Print and shaded views of the part. All mm, measured from the part's lowest x, y and z. Give positions to 0.01 mm unless a question says otherwise; leave off trailing zeros. Loops run counter-clockwise (first coordinate to the right, second up) from the corner with the lowest first, then second, coordinate; pieces in that order, holes last. Notation, with made-up numbers: (7.5, 79.5) - (12.5, 79.5) arc R24 cw to (12.5, 118.5) - close; hole circle Ø10 at (66.5, -38.75). An arc over 180 degrees is marked (long way). Return JSON: item names as keys, results as strings.
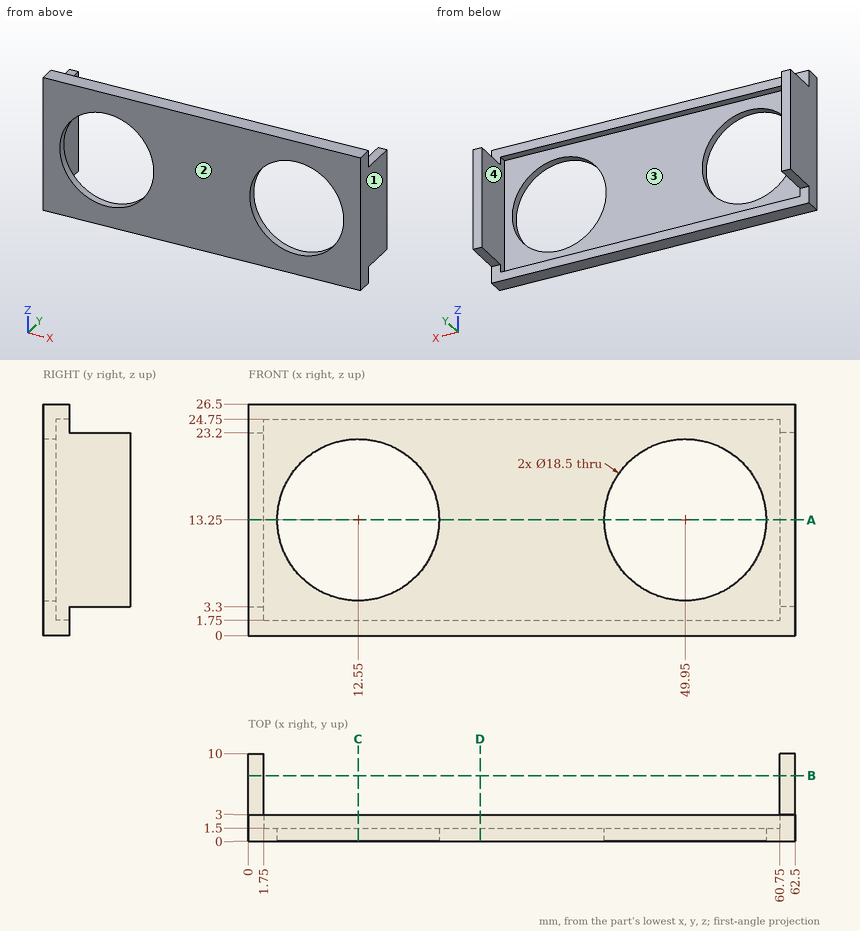
1. Drop flat-ended pins along their axis: P1, Ø5, axis at x = 24.5, z = 13.5, coming from the +Y side; P2, Ø1.7, axis at x = 31.5, z = 25.5, coming from the +Y side; P3, Ø0.9, axis at x = 61.5, y = 6.5, coming from the -Z side. Give the stop position or say it passes through.
Values follow:
{"P1": "stops at y = 1.5", "P2": "stops at y = 3", "P3": "stops at z = 3.3"}
2. Pull direction X, two halves, no side cores. Call the marked faces 1, 2, 3 and 4: +X half, -X half, draft (parallel to the pull), parting line (faces both ways), or undercut.
Values follow:
{"face 1": "+X half", "face 2": "draft", "face 3": "undercut", "face 4": "undercut"}
3. Cut at C-C, the plane x = 12.55. Write the cut outline in (y, z), plus the area to 4 significant figures.
Values follow:
{"outline": "(0, 0) - (3, 0) - (3, 1.75) - (1.5, 1.75) - (1.5, 4) - (0, 4) - close; (0, 22.5) - (1.5, 22.5) - (1.5, 24.75) - (3, 24.75) - (3, 26.5) - (0, 26.5) - close", "area": "17.25 mm²"}
4. Drill centre lines: probe 1 along X at (y, z) = (0.95, 13.25); probe 2 along X at (y, z) = (9, 21.5); probe 3 along Z at (x, y) = (33, 2). Where is each one in solid material? Low to high.
Values follow:
{"probe 1": "x = 0 to 3.3, 21.8 to 40.7, 59.2 to 62.5", "probe 2": "x = 0 to 1.75, 60.75 to 62.5", "probe 3": "z = 0 to 1.75, 24.75 to 26.5"}
5. Cut at B-B, the plane y = 7.5. Write the cut outline in (x, z), plus the area to 4 significant figures.
Values follow:
{"outline": "(0, 3.3) - (1.75, 3.3) - (1.75, 23.2) - (0, 23.2) - close; (60.75, 3.3) - (62.5, 3.3) - (62.5, 23.2) - (60.75, 23.2) - close", "area": "69.65 mm²"}
6. Cut at D-D, the plane x = 26.5. Write the cut outline in (y, z).
Values follow:
{"outline": "(0, 0) - (3, 0) - (3, 1.75) - (1.5, 1.75) - (1.5, 24.75) - (3, 24.75) - (3, 26.5) - (0, 26.5) - close"}
7. Cut at A-A, the plane z = 13.25. Write the cut outline in (x, y), plus the area to 3 significant figures.
Values follow:
{"outline": "(0, 0) - (3.3, 0) - (3.3, 1.5) - (1.75, 1.5) - (1.75, 10) - (0, 10) - close; (21.8, 0) - (40.7, 0) - (40.7, 1.5) - (21.8, 1.5) - close; (59.2, 0) - (62.5, 0) - (62.5, 10) - (60.75, 10) - (60.75, 1.5) - (59.2, 1.5) - close", "area": "68.0 mm²"}
